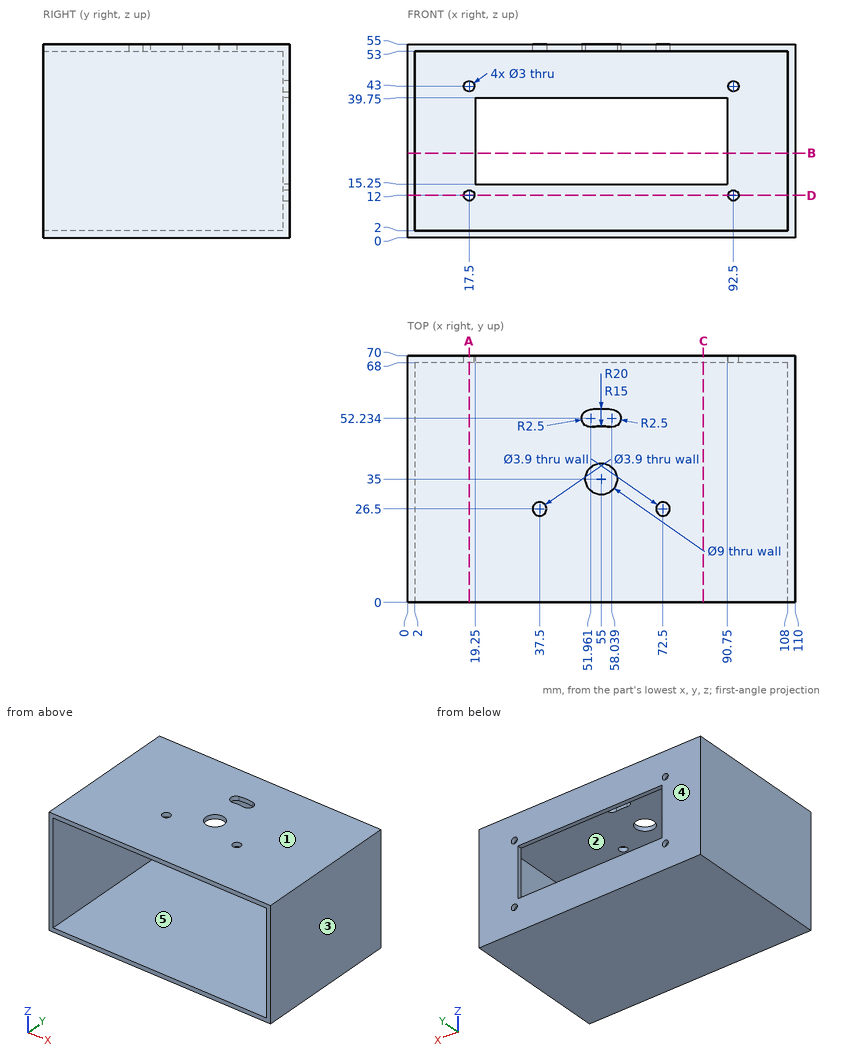
The figure shows three views and two pictorial views of one solid part (mm, origin at its lowest corner). Answer the questions. A direction names the side the tool comes from. Give positions to 0.01 mm unless a question says otherwise; leave off trailing zeros. Order: outer loops, then holes, each group sorted by start corner. A loop starts at its lowest first (then second) coordinate and runs counter-clockwise, first axis right, second up. Notation, with made-up numbers: (-40, 83.5) -> (10, 83.5) arc R21 ccw to (10, 110.5) -> close; hole circle Ø10 at (-12.5, 6.5). An arc over 180 degrees is marked (long way). One line per item, written item: value.
1) Find section C-C, the plane x = 84. Determine the outline of the cut face in (y, z), plus the area to 3 significant figures.
Reported:
outline: (0, 0) -> (70, 0) -> (70, 15.25) -> (68, 15.25) -> (68, 2) -> (0, 2) -> close; (0, 53) -> (68, 53) -> (68, 39.75) -> (70, 39.75) -> (70, 55) -> (0, 55) -> close
area: 333 mm^2
2) Find section D-D, the plane z = 12. Determine the outline of the cut face in (x, y).
Reported:
outline: (0, 0) -> (2, 0) -> (2, 68) -> (16, 68) -> (16, 70) -> (0, 70) -> close; (19, 68) -> (91, 68) -> (91, 70) -> (19, 70) -> close; (94, 68) -> (108, 68) -> (108, 0) -> (110, 0) -> (110, 70) -> (94, 70) -> close
3) Find the intervals of material crossed by line 1 (Z direction, x = 92.5, y = 68.65); line 2 (Y direction, x = 55, z = 54.5); line 3 (X direction, y = 35, z = 53.9), in increasing order.
Reported:
line 1: z = 0 to 10.5, 13.5 to 41.5, 44.5 to 55
line 2: y = 0 to 30.5, 39.5 to 50, 55 to 70
line 3: x = 0 to 50.5, 59.5 to 110
4) A tool of negligible diameter and unlimited length cuts with its end or side. For the marked faces 1 and 2, from which of +Z, -Z, +X, -X, +Y, -Y can it reach the whole face along a straight path? Write none if from no direction.
Reported:
face 1: +Z, +X, -X, +Y, -Y
face 2: -Y
5) Find section B-B, the plane z = 24. Determine the outline of the cut face in (x, y), plus the area to 3 significant figures.
Reported:
outline: (0, 0) -> (2, 0) -> (2, 68) -> (19.25, 68) -> (19.25, 70) -> (0, 70) -> close; (90.75, 68) -> (108, 68) -> (108, 0) -> (110, 0) -> (110, 70) -> (90.75, 70) -> close
area: 349 mm^2
6) Find section A-A, the plane x = 17.5. Determine the outline of the cut face in (y, z).
Reported:
outline: (0, 0) -> (70, 0) -> (70, 10.5) -> (68, 10.5) -> (68, 2) -> (0, 2) -> close; (0, 53) -> (68, 53) -> (68, 44.5) -> (70, 44.5) -> (70, 55) -> (0, 55) -> close; (68, 13.5) -> (70, 13.5) -> (70, 41.5) -> (68, 41.5) -> close
7) Flat-ended cylindrical pins translate along their axes: P1, Ø1.8, axis at x = 17.5, z = 43, coming from the +Y side; P2, Ø2.5, axis at x = 37.5, y = 26.5, coming from the +Z side; P3, Ø5, axis at x = 74, z = 49, coming from the -Y side. Find the tip coordinate at first contact, or state that the pin passes through.
Reported:
P1: passes through
P2: stops at z = 2
P3: stops at y = 68
8) Determine the mould class of the marked faces 3, 4 and 5 for opening direction X: pulls with the +X half, pulls with the -X half, needs draft (parallel to the pull), parting line crosses it, or undercut.
Reported:
face 3: pulls with the +X half
face 4: needs draft
face 5: undercut
